from build123d import *

# Parameters (mm, degrees)
BOSS_EXTRUDE1_DEPTH = 5.5


with BuildPart() as part:
    # Sketch1 → Boss-Extrude1 (new body)
    with BuildSketch(Plane.XY):
        with BuildLine():
            Line((-0.821374058, -0.5), (-3.968626967, -0.5))
            ThreePointArc((-3.968626967, -0.5), (0, -4), (3.968626967, -0.5))
            Line((3.968626967, -0.5), (0.821374058, -0.5))
            ThreePointArc((0.821374058, -0.5), (0, -0.961590008), (-0.821374058, -0.5))
        make_face()
        with BuildLine():
            ThreePointArc((-0.5, 3.968626967), (-2.828427125, 2.828427125), (-3.968626967, 0.5))
            Line((-3.968626967, 0.5), (-0.821374058, 0.5))
            ThreePointArc((-0.821374058, 0.5), (-0.679946815, 0.679946815), (-0.5, 0.821374058))
            Line((-0.5, 0.821374058), (-0.5, 3.968626967))
        make_face()
        with BuildLine():
            ThreePointArc((3.968626967, 0.5), (2.828427125, 2.828427125), (0.5, 3.968626967))
            Line((0.5, 3.968626967), (0.5, 0.821374058))
            ThreePointArc((0.5, 0.821374058), (0.679946815, 0.679946815), (0.821374058, 0.5))
            Line((0.821374058, 0.5), (3.968626967, 0.5))
        make_face()
        with BuildLine():
            Line((-0.821374058, 0.5), (-3.968626967, 0.5))
            ThreePointArc((-3.968626967, 0.5), (-4, 0), (-3.968626967, -0.5))
            Line((-3.968626967, -0.5), (-0.821374058, -0.5))
            ThreePointArc((-0.821374058, -0.5), (-0.961590008, 0), (-0.821374058, 0.5))
        make_face()
        with BuildLine():
            Line((0.821374058, -0.5), (3.968626967, -0.5))
            ThreePointArc((3.968626967, -0.5), (3.992149037, -0.25049165), (4, 0))
            ThreePointArc((4, 0), (3.992149037, 0.25049165), (3.968626967, 0.5))
            Line((3.968626967, 0.5), (0.821374058, 0.5))
            ThreePointArc((0.821374058, 0.5), (0.925872678, 0.259644234), (0.961590008, 0))
            ThreePointArc((0.961590008, 0), (0.925872678, -0.259644234), (0.821374058, -0.5))
        make_face()
        with BuildLine():
            ThreePointArc((0.5, 3.968626967), (0, 4), (-0.5, 3.968626967))
            Line((-0.5, 3.968626967), (-0.5, 0.821374058))
            ThreePointArc((-0.5, 0.821374058), (0, 0.961590008), (0.5, 0.821374058))
            Line((0.5, 0.821374058), (0.5, 3.968626967))
        make_face()
        with BuildLine():
            Line((-3.968626967, 0.5), (-4.75, 0.5))
            Line((-4.75, 0.5), (-4.75, -0.5))
            Line((-4.75, -0.5), (-3.968626967, -0.5))
            ThreePointArc((-3.968626967, -0.5), (-4, 0), (-3.968626967, 0.5))
        make_face()
        with BuildLine():
            ThreePointArc((4, 0), (3.992149037, -0.25049165), (3.968626967, -0.5))
            Line((3.968626967, -0.5), (4.75, -0.5))
            Line((4.75, -0.5), (4.75, 0.5))
            Line((4.75, 0.5), (3.968626967, 0.5))
            ThreePointArc((3.968626967, 0.5), (3.992149037, 0.25049165), (4, 0))
        make_face()
        with BuildLine():
            Line((-0.5, 4.75), (-0.5, 3.968626967))
            ThreePointArc((-0.5, 3.968626967), (0, 4), (0.5, 3.968626967))
            Line((0.5, 3.968626967), (0.5, 4.75))
            Line((0.5, 4.75), (-0.5, 4.75))
        make_face()
    extrude(amount=BOSS_EXTRUDE1_DEPTH)


solid = part.part
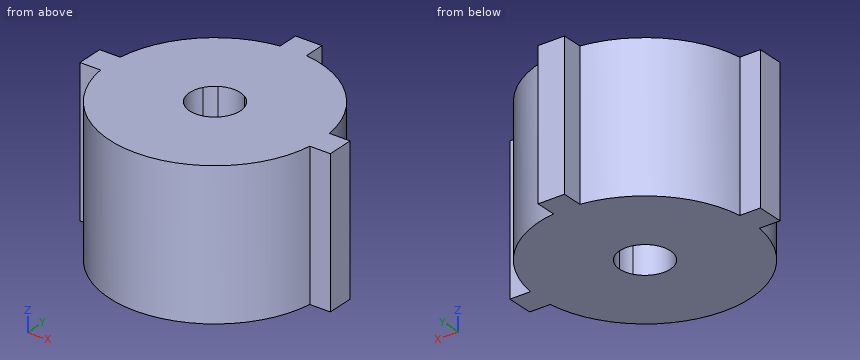
Can you work these out from the model? Positions are in its coordinate system, mm. Coordinates: 2 decimals unless noted, no trailing zeros. Write each loop counter-clockwise with the first axis right and the second up, starting at its lowest first coordinate (ties: lowest second). Pieces come first, ordered by that corner, then holes. Notation, with made-up numbers: (83, -2.5) - (91, -2.5) arc R27 ccw to (91, 35.5) - close; hole circle Ø4 at (-37, 85). An arc over 180 degrees is marked (long way). Return JSON: item names as keys, results as strings. Group by question number.
Item 1: Please list where these lines run through material, in increasing order: probe 1 along X at (y, z) = (4, 2.7); probe 2 along X at (y, z) = (0.75, 2.85).
Item 2: If we section it at A-A (z = 2.4): Write out the boundary of the cut face in (x, y), then the cut area to 3 significant figures.
Item 3: If we section it at C-C (x = 3.75): Write out the boundary of the cut face in (y, z).
Item 4: If we section it at D-D (y = 3.5): Write out the boundary of the cut face in (x, z).
Item 5: I'm going to push flat-ended pins straight in: pin 1 Ø0.9 at (y, z) = (4.5, 2) entering from -X; pin 2 Ø0.9 at (x, z) = (-4.5, 4) entering from +Y; pin 3 Ø3 at (x, z) = (-2.5, 2) entering from +Y. Where does each tip first touch, or does it pass through?
Item 6: If we section it at B-B (y = -0.25): Write out the boundary of the cut face in (x, z), then the cut area to 3 significant figures.
Return value:
{
 "1": {"probe 1": "x = -0.5 to 0.5", "probe 2": "x = -3.93 to -0.6, 0.6 to 3.93"},
 "2": {"outline": "(-4.75, -0.5) - (-3.97, -0.5) arc R4 ccw to (3.97, -0.5) - (4.75, -0.5) - (4.75, 0.5) - (3.97, 0.5) arc R4 ccw to (0.5, 3.97) - (0.5, 4.75) - (-0.5, 4.75) - (-0.5, 3.97) arc R4 ccw to (-3.97, 0.5) - (-4.75, 0.5) - close; hole circle Ø1.92 at (0, 0)", "area": "49.6 mm^2"},
 "3": {"outline": "(-1.39, 0) - (1.39, 0) - (1.39, 5.5) - (-1.39, 5.5) - close"},
 "4": {"outline": "(-1.94, 0) - (1.94, 0) - (1.94, 5.5) - (-1.94, 5.5) - close"},
 "5": {"pin 1": "stops at x = -0.5", "pin 2": "stops at y = 0.5", "pin 3": "stops at y = 3.87"},
 "6": {"outline": "(-4.75, 0) - (-0.93, 0) - (-0.93, 5.5) - (-4.75, 5.5) - close; (0.93, 0) - (4.75, 0) - (4.75, 5.5) - (0.93, 5.5) - close", "area": "42.0 mm^2"}
}
